Verification items for the finished model (mm, model axes). Face numbers are marked on the shaded views. A direction names the side the tool comes from. Coordinates: 2 decimals unless noted, no trailing zeros. Order: outer loops, then holes, each group sorted by start corner. A loop starts at its lowest first (then second) coordinate and runs counter-clockwise, first axis right, second up. Notation, with made-up numbers: (10, 1) -> (64, 1) arc R20 ccw to (64, 27) -> close; hole circle Ø3 at (-4, -2.75). An arc over 180 degrees is marked (long way). Write item = value, one per line. Start each with the question number.
1. Set-up check for the marked faces 1 and 2: record each of +Z, -Z, +X, -X, +Y, -Y from which the full face is reachable in a straight line by a thin tool's end or side.
2. Cross-section at A-A on z = 356.5. Record the cut outline in (x, y).
3. Thickness scan on line 1 along Z through (x, y) = (299, 538.5); line 2 along X through (y, z) = (489, 310.5); line 3 along Y through (x, z) = (105, 100). Record the ranges inside material, lowest first. Write a range as from..to.
4. Cross-section at C-C on y = 510. Record the cut outline in (x, z).
5. Go/stop test with flat-tipped pins: P1, Ø12, axis at x = 295, y = 418.5, coming from the -Z side; P2, Ø1, axis at x = 280.5, z = 314.5, coming from the +Y side. Record where each tip stops, or that it passes through.
6. Cross-section at B-B on x = 115. Record the cut outline in (y, z), plus the area to 3 significant figures.
7. Cross-section at D-D on y = 261.5. Record the cut outline in (x, z), plus the area to 3 significant figures.
from build123d import *

# Parameters (mm, degrees)
SKIZZE1_W                       = 400
SKIZZE1_H                       = 400
AUFSATZ_LINEAR_AUSTRAGEN1_DEPTH = 200
SKIZZE2_W                       = 400
SKIZZE2_H                       = 400
AUFSATZ_LINEAR_AUSTRAGEN2_DEPTH = 400
SKIZZE3_W                       = 400
SKIZZE3_H                       = 400
SCHNITT_LINEAR_AUSTRAGEN1_DEPTH = 1040.962535349


with BuildPart() as part:
    # Skizze1 → Aufsatz-Linear austragen1 (new body)
    with BuildSketch(Plane(origin=(0, 0, 0), x_dir=(1, 0, 0), z_dir=(0, 1, 0))):
        with Locations((200, -200)):
            Rectangle(SKIZZE1_W, SKIZZE1_H)
    extrude(amount=AUFSATZ_LINEAR_AUSTRAGEN1_DEPTH)

    # Skizze2 → Aufsatz-Linear austragen2 (add)
    with BuildSketch(Plane(origin=(0, 200, 0), x_dir=(1, 0, 0), z_dir=(0, 1, 0))):
        with Locations((200, -200)):
            Rectangle(SKIZZE2_W, SKIZZE2_H)
    extrude(amount=AUFSATZ_LINEAR_AUSTRAGEN2_DEPTH)

    # Skizze3 → Schnitt-Linear austragen1 (cut, through all, along a direction that is not the sketch's normal)
    with BuildSketch(Plane(origin=(0, 600, 0), x_dir=(1, 0, 0), z_dir=(0, 1, 0))):
        with Locations((200, -200)):
            Rectangle(SKIZZE3_W, SKIZZE3_H)
    extrude(amount=-SCHNITT_LINEAR_AUSTRAGEN1_DEPTH, dir=(-0.577350269, 0.577350269, -0.577350269), mode=Mode.SUBTRACT)


solid = part.part
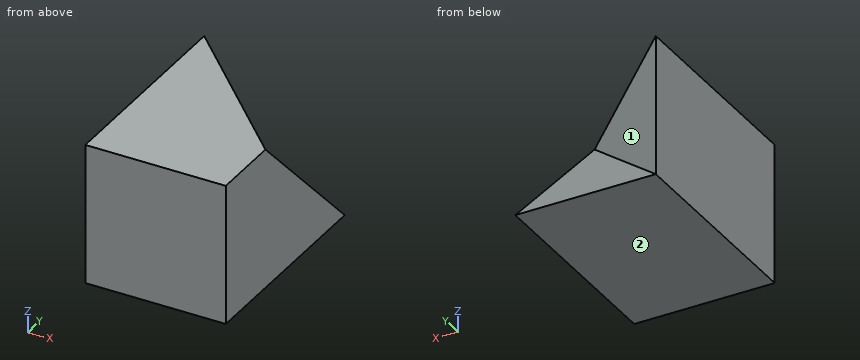
Worked out:
q1.face_1 = +Z, +X, +Y
q1.face_2 = -Z, +X, -X, +Y, -Y
q2.outline = (0, 0) -> (400, 0) -> (400, 243.5) -> (356.5, 243.5) -> (0, 600) -> close
q3.line_1 = 0..61.5
q3.line_2 = 0..111
q3.line_3 = 0..500
q4.outline = (0, 0) -> (400, 0) -> (400, 90) -> (90, 90) -> (90, 400) -> (0, 400) -> close
q5.P1 = 0
q5.P2 = 320
q6.outline = (0, 0) -> (600, 0) -> (485, 115) -> (485, 400) -> (0, 400) -> close
q6.area = 201,000 mm²
q7.outline = (0, 0) -> (400, 0) -> (400, 338.5) -> (338.5, 338.5) -> (338.5, 400) -> (0, 400) -> close
q7.area = 156,000 mm²
